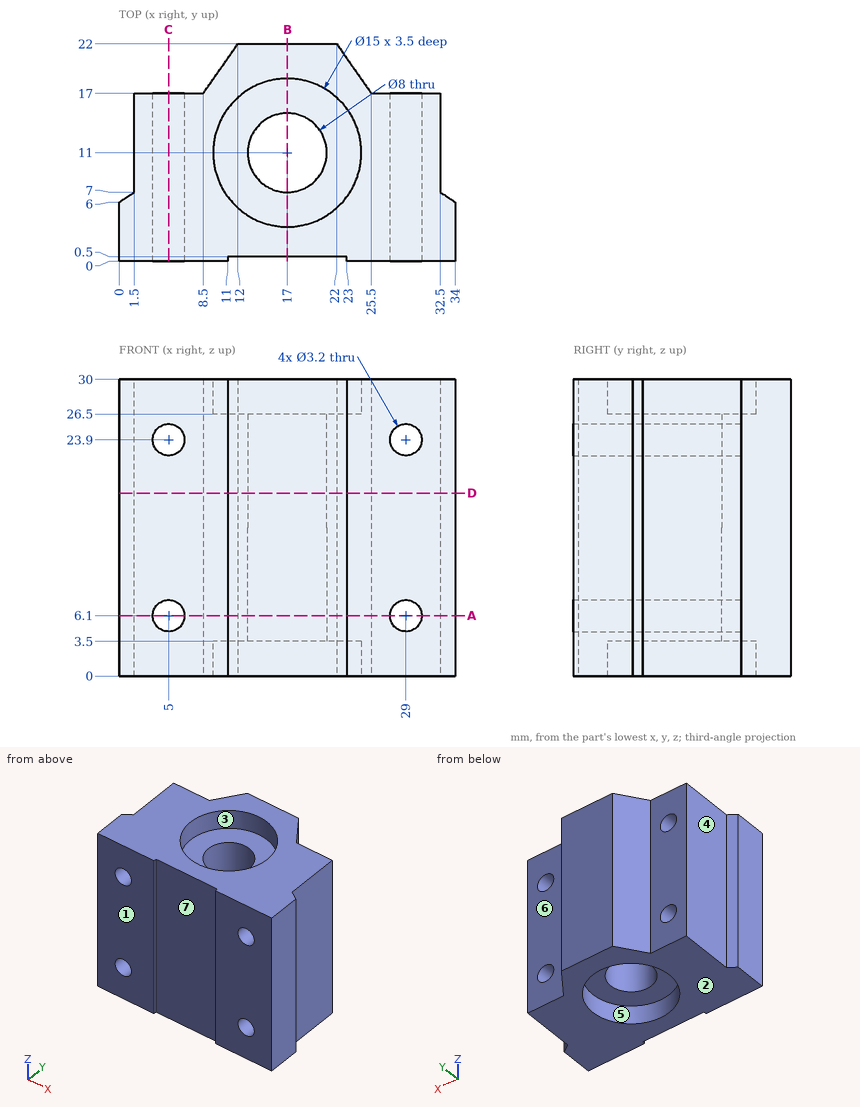
Design review of the part shown in the three views and the two pictorial views. Dimensions are in mm from the part's minimum x, y and z. A direction names the side the tool comes from. Round coordinates to 2 decimals unless told otherwise and drop trailing zeros. Order: outer loops, then holes, each group sorted by start corner. A loop starts at its lowest first (then second) coordinate and runs counter-clockwise, first axis right, second up. Notation, with made-up numbers: (-16.5, -28) -> (25.5, -28) arc R35 cw to (25.5, 5) -> close; hole circle Ø1 at (29, 72). An arc over 180 degrees is marked (long way). Write item = value, one per line. Start each with the question number.
1) Tool access review of the marked faces 4, 5, 6 and 7: name each direction out of +Z, -Z, +X, -X, +Y, -Y from which nothing blocks a thin tool from reaching the whole face with its end or side.
2) Take a section at D-D on z = 18.5. State the section outline as (x, y) points, plus the area to 3 significant figures.
3) To check wall thickness, follow line 1 (Z direction, x = 5, y = 7.5); line 2 (Y direction, x = 17, z = 2.15); line 3 (X direction, y = 10.75, z = 8.5). State the ranges of each line that lie inside material, in increasing order. Write a range as from..to.
4) Take a section at A-A on z = 6.1. State the section outline as (x, y) points, plus the area to 3 significant figures.
5) Take a section at C-C on x = 5. State the section outline as (y, z) points, plus the area to 3 significant figures.
6) Insertion check: pin 1 (1 mm diameter, centred on y = 10, z = 27, fed in from +X); pin 2 (3.5 mm diameter, centred on x = 30, z = 20.5, fed in from +Y); pin 3 (4 mm diameter, centred on y = 11, z = 7.5, fed in from -X). Each pin has a flat end and moves straight along its axis. Give the tip position at first contact, or say it passes through.
7) Take a section at B-B on x = 17. State the section outline as (y, z) points.
8) The part is to be moulded in two halves that separate along Y. For the marked faces 1, 2 and 3, say which applies: +Y half, -Y half, draft (parallel to the pull), parting line (faces both ways), or undercut.
Verdict:
q1.face_4 = +Z, -Z, -X, +Y
q1.face_5 = -Z
q1.face_6 = +Z, -Z, +X, +Y
q1.face_7 = +Z, -Z, -Y
q2.outline = (0, 0) -> (11, 0) -> (11, 0.5) -> (23, 0.5) -> (23, 0) -> (34, 0) -> (34, 6) -> (32.5, 7) -> (32.5, 17) -> (25.5, 17) -> (22, 22) -> (12, 22) -> (8.5, 17) -> (1.5, 17) -> (1.5, 7) -> (0, 6) -> close; hole circle Ø8 at (17, 11)
q2.area = 558 mm2
q3.line_1 = 0..4.5, 7.7..22.3, 25.5..30
q3.line_2 = 0.5..3.5, 18.5..22
q3.line_3 = 1.5..13.01, 20.99..32.5
q4.outline = (0, 0) -> (3.4, 0) -> (3.4, 17) -> (1.5, 17) -> (1.5, 7) -> (0, 6) -> close; (6.6, 0) -> (11, 0) -> (11, 0.5) -> (23, 0.5) -> (23, 0) -> (27.4, 0) -> (27.4, 17) -> (25.5, 17) -> (22, 22) -> (12, 22) -> (8.5, 17) -> (6.6, 17) -> close; (30.6, 0) -> (34, 0) -> (34, 6) -> (32.5, 7) -> (32.5, 17) -> (30.6, 17) -> close; hole circle Ø8 at (17, 11)
q4.area = 449 mm2
q5.outline = (0, 0) -> (17, 0) -> (17, 4.5) -> (0, 4.5) -> close; (0, 7.7) -> (17, 7.7) -> (17, 22.3) -> (0, 22.3) -> close; (0, 25.5) -> (17, 25.5) -> (17, 30) -> (0, 30) -> close
q5.area = 401 mm2
q6.pin_1 = 32.5
q6.pin_2 = 17
q6.pin_3 = 1.5
q7.outline = (0.5, 0) -> (3.5, 0) -> (3.5, 3.5) -> (7, 3.5) -> (7, 26.5) -> (3.5, 26.5) -> (3.5, 30) -> (0.5, 30) -> close; (15, 3.5) -> (18.5, 3.5) -> (18.5, 0) -> (22, 0) -> (22, 30) -> (18.5, 30) -> (18.5, 26.5) -> (15, 26.5) -> close
q8.face_1 = -Y half
q8.face_2 = draft
q8.face_3 = undercut
